Verification items for the finished model (mm, model axes). A direction names the side the tool comes from. Give positions to 0.01 mm unless a question says otherwise; leave off trailing zeros. Loops run counter-clockwise (first coordinate to the right, second up) from the corner with the lowest first, then second, coordinate; pieces in that order, holes last. Notation, with made-up numbers: (77, 84.25) -> (124, 84.25) arc R27 ccw to (124, 119.25) -> close; hole circle Ø2 at (6, 24.5). An arc over 180 degrees is marked (long way). Use one line per item in the form item = value. Start each with the question number.
from build123d import *

# Parameters (mm, degrees)
F0_R     = 25.4
F1_DEPTH = 6.35
F2_R     = 22.86
F3_DEPTH = 10.16
F4_R     = 22.86
F4_R_2   = 20.32
F4_R_3   = 14.8488227635
F5_DEPTH = 10.16
F6_R     = 25.4
F6_R_2   = 22.86
F7_DEPTH = 10.16
F8_R     = 1.651
F9_DEPTH = 6.35


with BuildPart() as f1:
    # F0 (on Top) → F1 (new body)
    with BuildSketch(Plane.XY):
        Circle(F0_R)
    extrude(amount=F1_DEPTH)

    # F2 (on face) → F3 (join)
    with BuildSketch(Plane.XY.offset(6.35)):
        Circle(F2_R)
    extrude(amount=F3_DEPTH)

    # F4 (on face) → F5 (cut)
    with BuildSketch(Plane.XY.offset(16.51)):
        Circle(F4_R)
        Circle(F4_R_2, mode=Mode.SUBTRACT)
        Circle(F4_R_2)
        with BuildLine():
            ThreePointArc((2.8200390162, 17.158628647), (13.2553445021, 11.254643452), (17.3888227635, 0))
            ThreePointArc((17.3888227635, 0), (-11.254643452, -13.2553445021), (-2.8200390162, 17.158628647))
            ThreePointArc((-2.8200390162, 17.158628647), (0, 17.3888227635), (2.8200390162, 17.158628647))
        make_face(mode=Mode.SUBTRACT)
        with BuildLine():
            ThreePointArc((-2.8200390162, 17.158628647), (-11.254643452, -13.2553445021), (17.3888227635, 0))
            ThreePointArc((17.3888227635, 0), (13.2553445021, 11.254643452), (2.8200390162, 17.158628647))
            Line((2.8200390162, 17.158628647), (-2.8200390162, 17.158628647))
        make_face()
        Circle(F4_R_3, mode=Mode.SUBTRACT)
        Circle(F4_R_3)
        Polygon((-10.4057336106, -9.5245266735), (-6.9533198674, -9.5704237527), (-2.3904008896, -12.8855784419), (-5.8428146328, -12.8396813627), align=None, mode=Mode.SUBTRACT)
        Polygon((-7.4583858915, -1.049800532), (-4.3231170224, -2.4959527766), (-1.5030780063, -7.380403632), (-4.6383468754, -5.9342513873), align=None, mode=Mode.SUBTRACT)
        Polygon((5.8428146328, -12.8396813627), (6.9533198674, -9.5704237527), (11.5162388451, -6.2552690636), (10.4057336106, -9.5245266735), align=None, mode=Mode.SUBTRACT)
        Polygon((4.6383468754, -5.9342513873), (4.3231170224, -2.4959527766), (7.1431560386, 2.3884980787), (7.4583858915, -1.049800532), align=None, mode=Mode.SUBTRACT)
        Polygon((-12.2739116821, 6.9532001517), (-11.2507078801, 3.6555765868), (-12.9935878417, -1.7084563782), (-14.0167916437, 1.5891671866), align=None, mode=Mode.SUBTRACT)
        Polygon((2.8200390162, 6.9840519193), (0, 4.9919055533), (-5.6400780323, 4.9919055533), (-2.8200390162, 6.9840519193), align=None, mode=Mode.SUBTRACT)
        Polygon((2.8200390162, 13.8218406978), (0, 11.8296943319), (-5.6400780323, 11.8296943319), (-2.8200390162, 13.8218406978), align=None, mode=Mode.SUBTRACT)
        Polygon((14.0167916437, 1.5891671866), (11.2507078801, 3.6555765868), (9.5078279185, 9.0196095519), (12.2739116821, 6.9532001517), align=None, mode=Mode.SUBTRACT)
        with BuildLine():
            Line((-2.8200390162, 17.158628647), (2.8200390162, 17.158628647))
            ThreePointArc((2.8200390162, 17.158628647), (0, 17.3888227635), (-2.8200390162, 17.158628647))
        make_face()
    extrude(amount=-F5_DEPTH, mode=Mode.SUBTRACT)

    # F6 (on face) → F7 (join)
    with BuildSketch(Plane.XY.offset(6.35)):
        Circle(F6_R)
        Circle(F6_R_2, mode=Mode.SUBTRACT)
    extrude(amount=F7_DEPTH)

    # F8 (on face) → F9 (cut, through all)
    with BuildSketch(Plane.XY.offset(6.35)):
        Circle(F8_R)
    extrude(amount=-F9_DEPTH, mode=Mode.SUBTRACT)


solid = f1.part
Item 1: Sectioned sample at B-B, the plane y = 0. Enter the section's corners in (x, z).
Item 2: Sectioned sample at C-C, the plane x = 18. Enter the section's corners in (y, z).
Item 3: Draft check along X on faces 3 (the flat face through (7.3, 0.69, 11.5)), 4 (the flat face through (6, -2, 16.51)). Enter one of: +X half, -X half, draft (parallel to the pull), parting line (faces both ways), or undercut.
Item 4: Material ranges on line 1 (Y direction, x = 0, z = 11.25); line 2 (Y direction, x = 12, z = 9.5); line 3 (Y direction, x = -7, z = 15), recorded low to high.
Item 5: Sectioned sample at A-A, the plane z = 15.5. State how many separate pieces and enclosed holes the cut face has, and give its area (3 significant figures).
Item 6: Gauge pin test, flat ends, axial feed: pin 1 Ø8 at (x, z) = (-16.5, 4.5) entering from +Y; pin 2 Ø4.5 at (x, z) = (1, 10.5) entering from +Y; pin 3 Ø6 at (x, z) = (-5.5, 6.5) entering from +Y. Record the tip position at first contact, or that the pin passes through.
Item 7: Sectioned sample at D-D, the plane z = 1.75. Enter the section's corners in (x, y), and give its area (3 significant figures).
Item 8: Tool access check on faces 1 (the flat face through (-1, 13, 16.51)), 2 (the flat face through (-11.77, 5.33, 11.5)). Record the directions out of +Z, -Z, +X, -X, +Y, -Y that give a thin tool (end or side, any length) a straight path to the whole face; none if there is none.
Outcome:
q1.outline = (-25.4, 0) -> (-1.65, 0) -> (-1.65, 6.35) -> (-12.44, 6.35) -> (-12.44, 16.51) -> (-13.52, 16.51) -> (-13.52, 6.35) -> (-22.86, 6.35) -> (-22.86, 16.51) -> (-25.4, 16.51) -> close; (1.65, 0) -> (25.4, 0) -> (25.4, 16.51) -> (22.86, 16.51) -> (22.86, 6.35) -> (7.36, 6.35) -> (7.36, 16.51) -> (5.76, 16.51) -> (5.76, 6.35) -> (1.65, 6.35) -> close
q2.outline = (-17.92, 0) -> (17.92, 0) -> (17.92, 16.51) -> (14.09, 16.51) -> (14.09, 6.35) -> (-14.09, 6.35) -> (-14.09, 16.51) -> (-17.92, 16.51) -> close
q3.face_3 = undercut
q3.face_4 = draft
q4.line_1 = -25.4 to -22.86, 4.99 to 6.98, 11.83 to 13.82, 22.86 to 25.4
q4.line_2 = -22.39 to -19.46, 3.1 to 7.16, 19.46 to 22.39
q4.line_3 = -24.42 to -21.76, -12 to -9.57, -1.84 to -1.26, 21.76 to 24.42
q5.separate_pieces = 9
q5.enclosed_holes = 1
q5.area = 475 mm^2
q6.pin_1 = 22.11
q6.pin_2 = 25.4
q6.pin_3 = 25.28
q7.outline = circle Ø50.8 at (0, 0); hole circle Ø3.3 at (0, 0)
q7.area = 2,020 mm^2
q8.face_1 = +Z, +X, -X, +Y, -Y
q8.face_2 = +Z
